Can you work these out from the drawing? Everything is in mm from the part's minimum corner. Give positions to 0.01 mm unless a question says otherwise; leave off trailing zeros. Order: outer loops, then holes, each group sorted by start corner. A loop starts at its lowest first (then second) coordinate and runs counter-clockwise, first axis right, second up. Notation, with made-up numbers: (-24.75, 63) - (34.25, 63) arc R33 cw to (34.25, 95) - close; hole circle Ø8 at (9.5, 50.5). An arc over 180 degrees is marked (long way). Write each question's results on one line, items separated by ' | '. Start each with the question number.
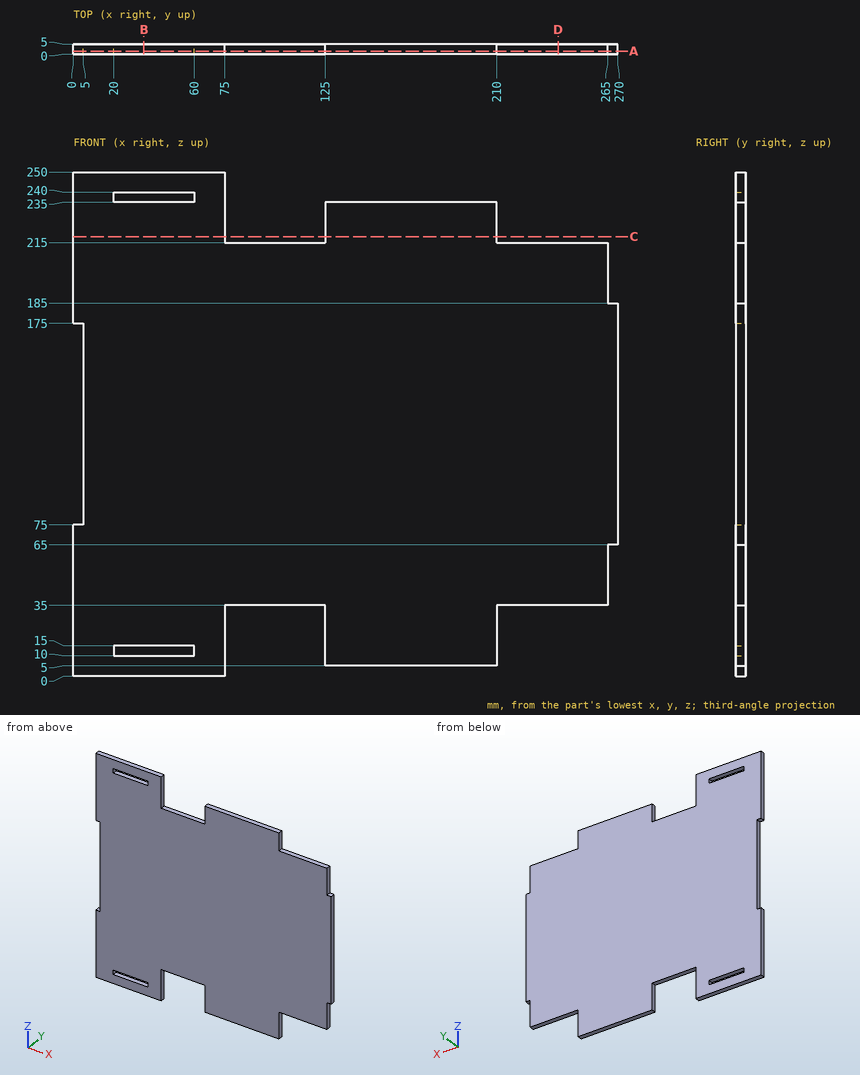
Q1. If we section it at D-D (x = 240.5): Please give me the cut outline in (y, z).
Q2. If we section it at A-A (y = 1.5): State how many separate pieces and enclosed holes the cut face has, plus the area to 3 significant figures.
Q3. If we section it at B-B (x = 35): Please give me the cut outline in (y, z), plus the area to 3 significant figures.
Q4. If we section it at C-C (z = 218): Please give me the cut outline in (x, y), plus the area to 3 significant figures.
Q5. Will these pins go through, and if not, where does the flat tip stop? P1, Ø2.5, axis at y = 3, z = 222.5, coming from the +X side; P2, Ø2.5, axis at y = 3.5, z = 44, coming from the +X side; P3, Ø1.5, axis at x = 267, y = 2, coming from the +Z side.
Q6. If I drill on probe 1 along Z at (x, y) = (44.5, 1.3); probe 2 along X at (y, z) = (0.4, 218); probe 3 along X at (y, z) = (3.9, 145), over which ranges is the centre line in solid material (lowest first)? Write a range as from..to.
Findings below:
1) outline: (0, 35) - (5, 35) - (5, 215) - (0, 215) - close
2) separate pieces: 1 | enclosed holes: 2 | area: 56,900 mm2
3) outline: (0, 0) - (5, 0) - (5, 10) - (0, 10) - close; (0, 15) - (5, 15) - (5, 235) - (0, 235) - close; (0, 240) - (5, 240) - (5, 250) - (0, 250) - close | area: 1,200 mm2
4) outline: (0, 0) - (75, 0) - (75, 5) - (0, 5) - close; (125, 0) - (210, 0) - (210, 5) - (125, 5) - close | area: 800 mm2
5) P1: stops at x = 210 | P2: stops at x = 265 | P3: stops at z = 185
6) probe 1: z = 0..10, 15..235, 240..250 | probe 2: x = 0..75, 125..210 | probe 3: x = 5..270
